Work out the finished part from the listing and answer in its coordinate system (mm). A direction names the side the tool comes from. Round coordinates to 2 decimals unless told otherwise and drop trailing zeros. Write each loop counter-clockwise with the first axis right and the second up, starting at its lowest first coordinate (ties: lowest second). Pieces come first, ordered by that corner, then holes.
1. Find section B-B (y = 0). Write down the section's boundary in (x, z) (3 decimals).
2. Find section A-A (x = 0). Write down the section's boundary in (y, z) (3 decimals), and give its area (3 significant figures).
3. Determine the mould class of faces 1 (the face through (0, 17, 12.7)), 2 (the face through (-3.827, -17.233, 34.436)), 3 (the face through (5, -16, 69.85)) for opening direction X: pulls with the +X half, pulls with the -X half, needs draft (parallel to the pull), parting line crosses it, or undercut.
4. Straight lines are drawn through the part: probe 1 along Y at (x, z) = (0, 48); probe 2 along Y at (x, z) = (0, 15) (3 decimals); probe 3 along X at (y, z) = (-9, 13). For each, find the intervals that lie inside material, in ascending order.
5. Find section D-D (z = 27.5). Write down the section's boundary in (x, y), and give its area (3 significant figures).
6. Flat-ended cylindrical pins translate along their axes: pin 1 Ø3 at (x, z) = (13.5, 29.5) entering from +Y; pin 2 Ø1.5 at (y, z) = (10.5, 16) entering from +X; pin 3 Ø4 at (y, z) = (7, 16.5) entering from -X. Find the tip coordinate at first contact, or state that the pin passes through.
7. Find section C-C (x = -9.5). Write down the section's boundary in (y, z) (3 decimals).
8. A tool of negligible diameter and unlimited length cuts with its end or side. For faces 4 (the face through (-16.51, -1, 6)), 5 (the face through (-17.076, 2.423, 9.272)), 6 (the face through (0, 3.175, 18)), 7 (the face through (-4.762, 12, 16)), 8 (the face through (-8, 7, 15.24)), from which of +Z, -Z, +X, -X, +Y, -Y can it reach the whole face along a straight path? Write none if from no direction.
```python
from build123d import *

# Parameters (mm, degrees)
F0_R      = 17.653
F0_R_2    = 16.383
F1_DEPTH  = 69.85
F2_W      = 12.7
F2_H      = 7.62
F6_R      = 2.54
F7_DEPTH  = 25.4
F8_R      = 15.875
F8_R_2    = 13.97
F9_DEPTH  = 2.54
F10_DEPTH = 7.62
F11_DEPTH = 2.54
F3_W      = 9.525
F3_H      = 5.08
F12_DEPTH = 25.4
F13_W     = 6.35
F13_H     = 5.588
F14_DEPTH = 16.51


with BuildPart() as f1:
    # F0 (on Top) → F1 (new body)
    with BuildSketch(Plane.XY):
        Circle(F0_R)
        Circle(F0_R_2, mode=Mode.SUBTRACT)
    extrude(amount=F1_DEPTH)

    # F2 (on Right) → F4 (join, up to the next surface of F1)
    with BuildSketch(Plane.YZ):
        with Locations((9.525, 16.51)):
            Rectangle(F2_W, F2_H)
    extrude(until=Until.NEXT, dir=(-1, 0, 0))

    # F2 (on Right) → F5 (join, up to the next surface of F1)
    with BuildSketch(Plane.YZ):
        with Locations((9.525, 16.51)):
            Rectangle(F2_W, F2_H)
    extrude(until=Until.NEXT)

    # F6 (on Right) → F7 (cut)
    with BuildSketch(Plane.YZ):
        with Locations((0, 8.509)):
            Circle(F6_R)
    extrude(amount=-F7_DEPTH, mode=Mode.SUBTRACT)

    # F8 (on face) → F9 (join)
    with BuildSketch(Plane(origin=(0, 0, 12.7), x_dir=(1, 0, 0), z_dir=(0, 0, -1))):
        Circle(F8_R)
        Circle(F8_R_2, mode=Mode.SUBTRACT)
    extrude(amount=-F9_DEPTH)

    # F8 (on face) → F10 (join)
    with BuildSketch(Plane(origin=(0, 0, 12.7), x_dir=(1, 0, 0), z_dir=(0, 0, -1))):
        Circle(F8_R)
        Circle(F8_R_2, mode=Mode.SUBTRACT)
    extrude(amount=-F10_DEPTH)

    # F8 (on face) → F11 (cut)
    with BuildSketch(Plane(origin=(0, 0, 12.7), x_dir=(1, 0, 0), z_dir=(0, 0, -1))):
        with BuildLine():
            Line((13.6044211564, -3.175), (-13.6044211564, -3.175))
            ThreePointArc((-13.6044211564, -3.175), (0, -13.97), (13.6044211564, -3.175))
        make_face()
    extrude(amount=-F11_DEPTH, mode=Mode.SUBTRACT)

    # F3 (on Front) → F12 (cut)
    with BuildSketch(Plane.XZ):
        with Locations((0, 15.24)):
            Rectangle(F3_W, F3_H)
    extrude(amount=-F12_DEPTH, mode=Mode.SUBTRACT)

    # F13 (on Right) → F14 (cut)
    with BuildSketch(Plane.YZ):
        with Locations((0, 8.509)):
            Rectangle(F13_W, F13_H)
    extrude(amount=-F14_DEPTH, mode=Mode.SUBTRACT)


solid = f1.part
```
Worked answers:
1. outline: (-17.653, 0) - (-16.383, 0) - (-16.383, 5.715) - (-16.51, 5.715) - (-16.51, 5.969) - (-17.653, 5.969) - close; (-17.653, 11.049) - (-16.51, 11.049) - (-16.51, 11.303) - (-16.383, 11.303) - (-16.383, 69.85) - (-17.653, 69.85) - close; (-15.875, 12.7) - (-13.97, 12.7) - (-13.97, 20.32) - (-15.875, 20.32) - close; (13.97, 12.7) - (15.875, 12.7) - (15.875, 20.32) - (13.97, 20.32) - close; (16.383, 0) - (17.653, 0) - (17.653, 69.85) - (16.383, 69.85) - close
2. outline: (-17.653, 0) - (-16.383, 0) - (-16.383, 69.85) - (-17.653, 69.85) - close; (-15.875, 12.7) - (-13.97, 12.7) - (-13.97, 20.32) - (-15.875, 20.32) - close; (3.175, 17.78) - (15.875, 17.78) - (15.875, 20.32) - (3.175, 20.32) - close; (16.383, 0) - (17.653, 0) - (17.653, 12.7) - (16.383, 12.7) - close; (16.383, 17.78) - (17.653, 17.78) - (17.653, 69.85) - (16.383, 69.85) - close
2. area: 218 mm2
3. face 1: undercut
3. face 2: parting line crosses it
3. face 3: needs draft
4. probe 1: y = -17.65 to -16.38, 16.38 to 17.65
4. probe 2: y = -17.653 to -16.383, -15.875 to -13.97
4. probe 3: x = -15.19 to -13.69, -13.08 to -10.68, 10.68 to 13.08, 13.69 to 15.19
5. outline: circle Ø35.31 at (0, 0); hole circle Ø32.77 at (0, 0)
5. area: 136 mm2
6. pin 1: stops at y = 12.95
6. pin 2: stops at x = 14.72
6. pin 3: stops at x = -16.93
7. outline: (-14.879, 0) - (-13.347, 0) - (-13.347, 69.85) - (-14.879, 69.85) - close; (-12.719, 12.7) - (-10.243, 12.7) - (-10.243, 20.32) - (-12.719, 20.32) - close; (3.175, 15.24) - (10.243, 15.24) - (10.243, 12.7) - (13.347, 12.7) - (13.347, 0) - (14.879, 0) - (14.879, 69.85) - (13.347, 69.85) - (13.347, 20.32) - (3.175, 20.32) - close
8. face 4: none
8. face 5: -X
8. face 6: +Z, -Z
8. face 7: +Y
8. face 8: -Z
